Design review of the part built by this model. Coordinates are the model's own, in mm. Coordinates: 2 decimals unless noted, no trailing zeros. Order: outer loops, then holes, each group sorted by start corner. A loop starts at its lowest first (then second) coordinate and runs counter-clockwise, first axis right, second up. Notation, with made-up numbers: (-5.75, 16.25) -> (33.25, 16.25) arc R16 cw to (33.25, 30.25) -> close; hole circle Ø7 at (5.5, 38.25). An arc over 180 degrees is marked (long way). Write item = value, one per line.
Autodesk Inventor part; units mm, degrees
ref_plane "YZ Plane" through (0, 0, 0) normal (1, 0, 0) x (0, 1, 0)
ref_plane "XZ Plane" through (0, 0, 0) normal (0, 1, 0) x (-1, 0, 0)
ref_plane "XY Plane" through (0, 0, 0) normal (0, 0, 1) x (1, 0, 0)
sketch "Sketch1" plane through (0, 0, 0) normal (0, 1, 0) x (-1, 0, 0)
  arc A0 (-29.9263, -13.9549) -> (29.9263, -13.9549) centre (0, 0) ccw
  arc A1 (-32.6452, -15.2227) -> (32.6452, -15.2227) centre (0, 0) ccw
  line L0 (54.2691, 0) -> (-55.7933, 0) construction
  line L1 (29.9263, -13.9549) -> (32.6452, -15.2227)
  line L2 (-29.9263, -13.9549) -> (-32.6452, -15.2227)
  dimension "d0" = 66.04
  dimension "d1" = 3
  dimension "d2" = 25
  dimension "d3" = 25
extrude "Extrusion1" add sketch "Sketch1" along normal blind 6
sketch "Sketch2" plane through (0, 0, 0) normal (0, -1, 0) x (1, 0, 0)
  arc A0 (-32.6452, -15.2227) -> (32.6452, -15.2227) centre (0, 0) ccw
  line L0 (2, -35.9644) -> (2, -44.9644)
  line L1 (2, -44.9644) -> (-2, -44.9644)
  line L2 (-2, -44.9644) -> (-2, -35.9644)
  dimension "d6" = 9
  dimension "d7" = 2
  dimension "d8" = 2
extrude "Extrusion2" add sketch "Sketch2" against normal blind 30
sketch "Sketch3" plane through (2, 0, -35.9644) normal (1, 0, 0) x (0, 0, -1)
  circle A0 centre (4.5, 24) radius 1.75
  line L0 (9, 0) -> (9, 30)
  line L1 (0, 30) -> (9, 30)
  line L2 (9, 0) -> (0, 0)
  point P0 (-35.9644, 0)
  dimension "d11" = 3.5
  dimension "d12" = 4.5
  dimension "d16" = 24
extrude "Extrusion3" cut sketch "Sketch3" against normal blind 26
sketch "Sketch5" plane through (0, 30, 0) normal (0, 1, 0) x (1, 0, 0)
  line L0 (-2, 44.9644) -> (-2, 35.9644)
  line L1 (-2, 35.9644) -> (-2, -19.0356)
  line L2 (-2, -19.0356) -> (2, -19.0356)
  line L3 (2, -19.0356) -> (2, 35.9644)
  arc A0 (2, 35.9644) -> (-2, 35.9644) centre (0, 0) ccw
  dimension "d22" = 55
extrude "Extrusion5" add sketch "Sketch5" against normal blind 5
sketch "Sketch6" plane through (2, 0, -35.9644) normal (1, 0, 0) x (0, 0, -1)
  point P0 (-35.9644, 0)
properties part number "_3DPrint"
(1) We need section D-D (z = -40). Write out the cut boundary in (x, y), and give its area (3 significant figures).
Report:
outline = (-2, 0) -> (2, 0) -> (2, 22.31) -> (-2, 22.31) -> close; (-2, 25.69) -> (2, 25.69) -> (2, 30) -> (-2, 30) -> close
area = 107 mm²
(2) For L1, parallel to Y at x = 1, z = 7; L2, parallel to X at y = 3.5, z = -14.5; L3, parallel to X at y = 3.75, z = -20.5, list the stretches that pass through material, from the lowest coordinate up.
Report:
L1 = 25 to 30
L2 = -31.1 to -29.67, 29.67 to 31.1
L3 = -29.62 to -25.89, 25.89 to 29.62
(3) The part is to be moulded in two halves that separate along Y. For faces 1 (the flat face through (0, 0, -34)), 2 (the flat face through (-2, 26, -23)), 3 (the cylindrical face through (0.03, 25.18, -39.17)), 4 (the cylindrical face through (-0.03, 15.37, -36.02)), say which applies: released by +Y, released by -Y, zero draft, split by the parting line, or undercut.
Report:
face_1 = released by -Y
face_2 = zero draft
face_3 = undercut
face_4 = undercut
(4) We need section A-A (y = 24). Write out the cut boundary in (x, z), and give its area (3 significant figures).
Report:
outline = (-2, -44.96) -> (2, -44.96) -> (2, -42.21) -> (-2, -42.21) -> close; (-2, -38.71) -> (2, -38.71) -> (2, -35.96) arc R36.02 cw to (-2, -35.96) -> close
area = 21.9 mm²
(5) We need section B-B (z = -22.5). Write out the cut boundary in (x, y).
Report:
outline = (-28.13, 0) -> (-24.17, 0) -> (-24.17, 6) -> (-28.13, 6) -> close; (-2, 25) -> (2, 25) -> (2, 30) -> (-2, 30) -> close; (24.17, 0) -> (28.13, 0) -> (28.13, 6) -> (24.17, 6) -> close
(6) Insertion check: pin 1 (4.5 mm diameter, centred on y = 24, z = -40.46, fed in from -X); pin 2 (4 mm diameter, centred on y = 3.5, z = -38, fed in from +X); pin 3 (17.5 mm diameter, centred on x = 15.5, z = -23.5, fed in from +Y). Each pin has a flat end and moves straight along its axis. Give the tip position at first contact, or say it passes through.
Report:
pin_1 = -2
pin_2 = 2
pin_3 = 6
(7) We need section C-C (y = 3.75). Write out the cut boundary in (x, z), and give its area (3 significant figures).
Report:
outline = (-32.65, -15.22) arc R36.02 ccw to (-2, -35.96) -> (-2, -44.96) -> (2, -44.96) -> (2, -35.96) arc R36.02 ccw to (32.65, -15.22) -> (29.93, -13.95) arc R33.02 cw to (-29.93, -13.95) -> close
area = 271 mm²
